Input: part model. Units: mm. Frame: model coordinates. A direction names the side the tool comes from. Round coordinates to 2 decimals unless told otherwise and drop trailing zeros. Write each loop counter-clockwise with the first axis right and the second up, starting at its lowest first coordinate (ties: lowest second). Pieces come first, ordered by that corner, then holes. Notation, with made-up numbers: (-13.75, 46) -> (6.25, 46) arc R30 cw to (6.25, 83) -> close; hole circle Ø10 at (-2, -30.5). An arc over 180 degrees is marked (long way). Write item = value, one per line. Start each with the question number.
```python
from build123d import *

# Parameters (mm, degrees)
BOSS_EXTRUDE1_DEPTH                                 = 22
SKETCH2_R                                           = 35
CUT_EXTRUDE1_DEPTH                                  = 18
SKETCH3_R                                           = 14
BOSS_EXTRUDE2_DEPTH                                 = 7
FILLET1_R                                           = 4
SKETCH4_R                                           = 10
CUT_EXTRUDE2_DEPTH                                  = 83.953300115
CHAMFER1_SIZE                                       = 2
M8X1_25_TAPPED_HOLE1_D                              = 6.8
M8X1_25_TAPPED_HOLE1_DEPTH                          = 29.75
M8X1_25_TAPPED_HOLE1_CSINK_D                        = 8.05
M8X1_25_TAPPED_HOLE1_CSINK_ANGLE                    = 90
M8X1_25_TAPPED_HOLE1_TIP                            = 2.042926105
CIRPATTERN1_COUNT                                   = 6
CSK_FOR_M8_COUNTERSUNK_FLAT_HEAD_SCREW1_D           = 6
CSK_FOR_M8_COUNTERSUNK_FLAT_HEAD_SCREW1_DEPTH       = 20
CSK_FOR_M8_COUNTERSUNK_FLAT_HEAD_SCREW1_CSINK_D     = 8
CSK_FOR_M8_COUNTERSUNK_FLAT_HEAD_SCREW1_CSINK_ANGLE = 90
CSK_FOR_M8_COUNTERSUNK_FLAT_HEAD_SCREW1_TIP         = 1.802581857


with BuildPart() as part:
    # Sketch1 → Boss-Extrude1 (new body)
    with BuildSketch(Plane.XY):
        with BuildLine():
            Line((-50, -59.5), (50, -59.5))
            Line((50, -59.5), (50, -49.5))
            Line((50, -49.5), (34, -49.5))
            ThreePointArc((34, -49.5), (31.171572875, -48.328427125), (30, -45.5))
            Line((30, -45.5), (30, -41.306779105))
            ThreePointArc((30, -41.306779105), (30.792252789, -37.405831617), (33.043478261, -34.122991434))
            ThreePointArc((33.043478261, -34.122991434), (47.217043986, -5.176944775), (39.652173913, 26.152535326))
            ThreePointArc((39.652173913, 26.152535326), (38.421945373, 28.784159388), (38, 31.658332237))
            Line((38, 31.658332237), (38, 47.5))
            Line((38, 47.5), (0, 47.5))
            ThreePointArc((0, 47.5), (-44.028922841, 17.824251834), (-33.043478261, -34.122991434))
            ThreePointArc((-33.043478261, -34.122991434), (-30.792252789, -37.405831617), (-30, -41.306779105))
            Line((-30, -41.306779105), (-30, -45.5))
            ThreePointArc((-30, -45.5), (-31.171572875, -48.328427125), (-34, -49.5))
            Line((-34, -49.5), (-50, -49.5))
            Line((-50, -49.5), (-50, -59.5))
        make_face()
    extrude(amount=BOSS_EXTRUDE1_DEPTH)

    # Sketch2 → Cut-Extrude1 (cut)
    with BuildSketch(Plane.XY.offset(22)):
        Circle(SKETCH2_R)
    extrude(amount=-CUT_EXTRUDE1_DEPTH, mode=Mode.SUBTRACT)

    # Sketch3 → Boss-Extrude2 (add)
    with BuildSketch(Plane(origin=(0, 0, 0), x_dir=(-1, 0, 0), z_dir=(0, 0, -1))):
        with Locations(Location((0, 0, 0), (0, 0, 180))):
            Circle(SKETCH3_R)
    extrude(amount=BOSS_EXTRUDE2_DEPTH)

    # Fillet1
    fillet1_edges = [part.edges().sort_by_distance(p)[0] for p in [
        (-14, 0, 0),
    ]]
    fillet(fillet1_edges, radius=FILLET1_R)

    # Sketch4 → Cut-Extrude2 (cut, through all)
    with BuildSketch(Plane(origin=(0, 0, -7), x_dir=(-1, 0, 0), z_dir=(0, 0, -1))):
        Circle(SKETCH4_R)
    extrude(amount=-CUT_EXTRUDE2_DEPTH, mode=Mode.SUBTRACT)

    # Chamfer1
    chamfer1_edges = [part.edges().sort_by_distance(p)[0] for p in [
        (50, -54.5, 0),
        (-50, -54.5, 0),
        (-50, -54.5, 22),
        (50, -54.5, 22),
    ]]
    chamfer(chamfer1_edges, length=CHAMFER1_SIZE)

    # M8x1.25 Tapped Hole1
    with Locations(Plane(origin=(0, 47.5, 0), x_dir=(1, 0, 0), z_dir=(0, 1, 0))):
        with Locations((30.22415, -10.919516186)):
            CounterSinkHole(M8X1_25_TAPPED_HOLE1_D / 2, M8X1_25_TAPPED_HOLE1_CSINK_D / 2, depth=M8X1_25_TAPPED_HOLE1_DEPTH, counter_sink_angle=M8X1_25_TAPPED_HOLE1_CSINK_ANGLE)
            with Locations((0, 0, -(M8X1_25_TAPPED_HOLE1_DEPTH + M8X1_25_TAPPED_HOLE1_TIP / 2))):  # 118° drill point
                Cone(0, M8X1_25_TAPPED_HOLE1_D / 2, M8X1_25_TAPPED_HOLE1_TIP, mode=Mode.SUBTRACT)

    # Sketch10 → M6x1.0 Tapped Hole1 (revolve, cut)
    with BuildSketch(Plane(origin=(0, 39.887207207, 22), x_dir=(0, -1, 0), z_dir=(1, 0, 0))):
        Polygon((0, 0), (0, 16.502151548), (2.5, 15), (2.5, 0.525), (3.025, 0), align=None)
    m6x1_0_tapped_hole1 = revolve(axis=Axis((0, 39.887207207, 28.35), (0, 0, -1)), mode=Mode.SUBTRACT)

    # CirPattern1: M6x1.0 Tapped Hole1 ×6 about axis
    cirpattern1_axis = Axis((0, 0, 0), (0, 0, 1))
    for i in range(1, CIRPATTERN1_COUNT):
        add(m6x1_0_tapped_hole1.rotate(cirpattern1_axis, i * 360 / CIRPATTERN1_COUNT), mode=Mode.SUBTRACT)

    # CSK for M8 Countersunk Flat Head Screw1
    with Locations(Plane(origin=(0, -59.5, 0), x_dir=(-1, 0, 0), z_dir=(0, -1, 0))):
        with Locations((42, -11), (-42, -11)):
            CounterSinkHole(CSK_FOR_M8_COUNTERSUNK_FLAT_HEAD_SCREW1_D / 2, CSK_FOR_M8_COUNTERSUNK_FLAT_HEAD_SCREW1_CSINK_D / 2, depth=CSK_FOR_M8_COUNTERSUNK_FLAT_HEAD_SCREW1_DEPTH, counter_sink_angle=CSK_FOR_M8_COUNTERSUNK_FLAT_HEAD_SCREW1_CSINK_ANGLE)
            with Locations((0, 0, -(CSK_FOR_M8_COUNTERSUNK_FLAT_HEAD_SCREW1_DEPTH + CSK_FOR_M8_COUNTERSUNK_FLAT_HEAD_SCREW1_TIP / 2))):  # 118° drill point
                Cone(0, CSK_FOR_M8_COUNTERSUNK_FLAT_HEAD_SCREW1_D / 2, CSK_FOR_M8_COUNTERSUNK_FLAT_HEAD_SCREW1_TIP, mode=Mode.SUBTRACT)


solid = part.part
```
1. Mould query, pull axis X, two halves, no side actions, for faces 6 (the flat face through (40, -49.5, 8)), 7 (the flat face through (-50, -54, 11)), 8 (the conical face through (-34.93, 20.14, 5.76)). Classes: pulls with the +X half, pulls with the -X half, needs draft (parallel to the pull), parting line crosses it, or undercut.
2. Reachability of faces 1 (the cylindrical face through (47.165, -5.634, 10.846)), 2 (the cylindrical face through (0.96, 37.58, 14.34)), 3 (the flat face through (-30, -43, 11)), 4 (the flat face through (21, -29, 22)), 5 (the cylindrical face through (-45, -54, 11)) from +Z, -Z, +X, -X, +Y, -Y: full face, straight path, thin tool, end or side. Return the list, or none.
3. Section B-B (x = -42). Output: boundary loops of the cut face in (y, z).
4. Section A-A (y = 0). Output: boundary loops of the cut face in (x, z), then the cut area to 3 significant figures.
5. Pin query (flat end, axial travel): P1, Ø5.5, axis at x = 30.22, z = 10.92, coming from the +Y side; P2, Ø1.5, axis at y = -11, z = 13, coming from the +X side; P3, Ø4, axis at x = 34.54, y = -19.94, coming from the -Z side. Return the tip coordinate at first contact, or that it passes through.
6. Line query: line 1 along Y through (x, z) = (-35.5, 9); line 2 along Y through (x, z) = (-36, 16.75); line 3 along X through (y, z) = (-54.5, 13.75). Output: solid intervals per line, ascending.
Check sheet entries:
q1.face_6 = needs draft
q1.face_7 = pulls with the -X half
q1.face_8 = undercut
q2.face_1 = +Z, -Z, +X
q2.face_2 = +Z
q2.face_3 = +Z, -Z, -X
q2.face_4 = +Z, +X, -X, +Y, -Y
q2.face_5 = -Y
q3.outline = (-59.5, 0) -> (-49.5, 0) -> (-49.5, 8) -> (-58.5, 8) -> (-59.5, 7) -> close; (-59.5, 15) -> (-58.5, 14) -> (-49.5, 14) -> (-49.5, 22) -> (-59.5, 22) -> close; (-22.19, 0) -> (22.19, 0) -> (22.19, 22) -> (-22.19, 22) -> close
q4.outline = (-47.5, 0) -> (-18, 0) arc R4 cw to (-14, -4) -> (-14, -7) -> (-10, -7) -> (-10, 4) -> (-35, 4) -> (-35, 22) -> (-47.5, 22) -> close; (10, -7) -> (14, -7) -> (14, -4) arc R4 cw to (18, 0) -> (47.5, 0) -> (47.5, 22) -> (35, 22) -> (35, 4) -> (10, 4) -> close
q4.area = 813 mm2
q5.P1 = 17.36
q5.P2 = 46.38
q5.P3 = 0
q6.line_1 = -59.5 to -49.5, -31.56 to -22.25, -17.63 to 17.63, 22.25 to 31.56
q6.line_2 = -59.5 to -49.5, -30.99 to -21.98, -17.91 to 17.91, 21.98 to 30.99
q6.line_3 = -50 to -43.2, -40.8 to 40.8, 43.2 to 50
